Part model, mm, in its own coordinate system. A direction names the side the tool comes from. Coordinates: 2 decimals unless noted, no trailing zeros. Write each loop counter-clockwise with the first axis right and the second up, starting at its lowest first coordinate (ties: lowest second). Pieces come first, ordered by that corner, then holes. Notation, with made-up numbers: (70, 82) - (114, 82) arc R21 cw to (114, 95) - close; hole circle Ø2 at (11.5, -22.75). An arc over 180 degrees is marked (long way). Write each question's results on one line, items separated by ' | '.
from build123d import *

# Parameters (mm, degrees)
BOSS_EXTRU_1_DEPTH      = 50
CONG_1_R                = 3
COQUE2_START            = 3
COQUE2_DEPTH            = 47
ESQUISSE2_W             = 40
ESQUISSE2_H             = 8
ESQUISSE2_R             = 1.5
ESQUISSE2_W_2           = 8
ESQUISSE2_H_2           = 50
ESQUISSE2_W_3           = 25
BOSS_EXTRU_3_DEPTH      = 42
ESQUISSE3_W             = 36
ESQUISSE3_H             = 25
ENL_V_MAT_EXTRU_1_DEPTH = 10
ESQUISSE5_R             = 6.5
ENL_V_MAT_EXTRU_2_DEPTH = 10
ESQUISSE6_R             = 5.5
ENL_V_MAT_EXTRU_3_DEPTH = 10
ESQUISSE7_W             = 12
ESQUISSE7_H             = 12
ENL_V_MAT_EXTRU_4_DEPTH = 10


# Read off the part's stored shape, not the designer's step: Coque2
with BuildPart() as part:
    # Esquisse1 → Boss.-Extru.1 (new body)
    with BuildSketch(Plane(origin=(0, 0, 0), x_dir=(0, 0, -1), z_dir=(1, 0, 0))):
        Polygon((0, 0), (70, 0), (70, 140), (120, 140), (120, 230), (-30, 230), (-30, 140), (0, 140), align=None)
    extrude(amount=BOSS_EXTRU_1_DEPTH)

    # Congé1
    cong_1_edges = [part.edges().sort_by_distance(p)[0] for p in [
        (0, 140, -95),
        (0, 70, -70),
        (0, 0, -35),
        (0, 70, 0),
        (50, 70, -70),
        (25, 140, 0),
        (25, 140, 30),
        (25, 230, 30),
        (25, 230, -120),
        (25, 140, -120),
        (25, 140, -70),
        (25, 0, -70),
        (25, 0, 0),
        (50, 140, -95),
        (50, 185, -120),
        (50, 230, -45),
        (50, 185, 30),
        (50, 140, 15),
        (50, 70, 0),
        (0, 140, 15),
        (50, 0, -35),
        (0, 185, 30),
        (0, 230, -45),
        (0, 185, -120),
    ]]
    fillet(cong_1_edges, radius=CONG_1_R)

    # Coque2 outline → Coque2 (cut)
    with BuildSketch(Plane.YZ.offset(COQUE2_START)):
        with BuildLine():
            Line((137, -3), (3, -3))
            Line((3, -3), (3, -67))
            Line((3, -67), (137, -67))
            ThreePointArc((137, -67), (141.242640687, -68.757359313), (143, -73))
            Line((143, -73), (143, -117))
            Line((143, -117), (227, -117))
            Line((227, -117), (227, 27))
            Line((227, 27), (143, 27))
            Line((143, 27), (143, 3))
            ThreePointArc((143, 3), (141.242640687, -1.242640687), (137, -3))
        make_face()
    extrude(amount=COQUE2_DEPTH, mode=Mode.SUBTRACT)

    # Esquisse2 → Boss.-Extru.3 (add)
    # profile 1 of 4: a face of its own
    with BuildSketch(Plane(origin=(3, 0, 0), x_dir=(0, 0, -1), z_dir=(1, 0, 0))):
        with Locations((65, 223)):
            Rectangle(ESQUISSE2_W, ESQUISSE2_H)
        with Locations(Location((65, 223, 0), (0, 0, 180))):
            Circle(ESQUISSE2_R, mode=Mode.SUBTRACT)
    # profile 2 of 4: a face of its own
    with BuildSketch(Plane(origin=(3, 0, 0), x_dir=(0, 0, -1), z_dir=(1, 0, 0))):
        with Locations((7, 60)):
            Rectangle(ESQUISSE2_W_2, ESQUISSE2_H_2)
        with Locations(Location((7, 60, 0), (0, 0, 180))):
            Circle(ESQUISSE2_R, mode=Mode.SUBTRACT)
    # profile 3 of 4: a face of its own
    with BuildSketch(Plane(origin=(3, 0, 0), x_dir=(0, 0, -1), z_dir=(1, 0, 0))):
        with Locations((63, 60)):
            Rectangle(ESQUISSE2_W_2, ESQUISSE2_H_2)
        with Locations(Location((63, 60, 0), (0, 0, 180))):
            Circle(ESQUISSE2_R, mode=Mode.SUBTRACT)
    # profile 4 of 4: a face of its own
    with BuildSketch(Plane(origin=(3, 0, 0), x_dir=(0, 0, -1), z_dir=(1, 0, 0))):
        with Locations((25, 7)):
            Rectangle(ESQUISSE2_W_3, ESQUISSE2_H)
        with Locations(Location((25, 7, 0), (0, 0, 180))):
            Circle(ESQUISSE2_R, mode=Mode.SUBTRACT)
    extrude(amount=BOSS_EXTRU_3_DEPTH)

    # Esquisse3 → Enlèv. mat.-Extru.1 (cut)
    with BuildSketch(Plane.XY.offset(30)):
        with Locations((25, 195)):
            Rectangle(ESQUISSE3_W, ESQUISSE3_H)
    extrude(amount=-ENL_V_MAT_EXTRU_1_DEPTH, mode=Mode.SUBTRACT)

    # Esquisse5 → Enlèv. mat.-Extru.2 (cut)
    with BuildSketch(Plane.XY.offset(30)):
        with Locations((26, 161)):
            Circle(ESQUISSE5_R)
    extrude(amount=-ENL_V_MAT_EXTRU_2_DEPTH, mode=Mode.SUBTRACT)

    # Esquisse6 → Enlèv. mat.-Extru.3 (cut)
    with BuildSketch(Plane(origin=(0, 0, -70), x_dir=(-1, 0, 0), z_dir=(0, 0, -1))):
        with Locations((-25, 93)):
            Circle(ESQUISSE6_R)
    extrude(amount=-ENL_V_MAT_EXTRU_3_DEPTH, mode=Mode.SUBTRACT)

    # Esquisse7 → Enlèv. mat.-Extru.4 (cut)
    with BuildSketch(Plane(origin=(0, 0, -120), x_dir=(-1, 0, 0), z_dir=(0, 0, -1))):
        with Locations((-25, 184.5)):
            Rectangle(ESQUISSE7_W, ESQUISSE7_H)
    extrude(amount=-ENL_V_MAT_EXTRU_4_DEPTH, mode=Mode.SUBTRACT)


solid = part.part
(1) Saw through at C-C on x = 25. Count the separate pieces of the cut face and the enclosed holes in it, then the cut area to 3 significant figures.
Return value:
separate pieces: 4 | enclosed holes: 4 | area: 3,330 mm^2
(2) Saw through at A-A on y = 93. Write the cut outline in (x, z), then the cut area to 3 significant figures.
Return value:
outline: (0, -67) arc R3 ccw to (3, -70) - (19.5, -70) - (19.5, -67) - (3, -67) - (3, -3) - (50, -3) arc R3 ccw to (47, 0) - (3, 0) arc R3 ccw to (0, -3) - close; (30.5, -70) - (47, -70) arc R3 ccw to (50, -67) - (30.5, -67) - close | area: 451 mm^2
(3) Wall check: line 1 (Z direction, x = 30, y = 60); line 2 (Y direction, x = 19, z = -25); line 3 (Z direction, x = 24, y = 7). Give the ranges that are in metal, low to high. Write a range as from..to.
Return value:
line 1: z = -70..-64.5, -61.5..-59, -11..-8.5, -5.5..0 | line 2: y = 0..5.5, 8.5..11, 227..230 | line 3: z = -70..-67, -37.5..-26.5, -23.5..-12.5, -3..0
(4) 3-axis set-ups, long thin cutter, end or side, ignore diameter. For faces 5 (the flat face through (25, 140, -95)), 6 (the cylindrical face through (24.591, 154.655, 28.521)), 7 (the flat face through (24, 85, -7)): which of +Z, -Z, +X, -X, +Y, -Y reach the whole face in a straight line?
Return value:
face 5: -Z, +X, -X, -Y | face 6: +Z | face 7: +X
(5) Flat gauge pins, fed straight in: P1, Ø9, axis at x = 25, y = 93, coming from the -Z side; P2, Ø2, axis at x = 8, y = 43.5, coming from the -Z side; P3, Ø4, axis at x = 27, y = 9, coming from the +Z side. Where does each tip first touch, or does it go through?
Return value:
P1: stops at z = -3 | P2: stops at z = -70 | P3: stops at z = 0
(6) Two-plate mould, pull along Z, no slides. Class faces 1 (the flat face through (25, 176, 30)), 2 (the flat face through (26, 143, 15)), 3 (the flat face through (25, 69, -70)), 4 (the flat face through (0, 141, -44)): released by +Z, released by -Z, zero draft, split by the parting line, or undercut.
Return value:
face 1: released by +Z | face 2: undercut | face 3: released by -Z | face 4: zero draft
(7) Saw through at B-B on z = -93. Write the cut outline in (x, y), then the cut area to 3 significant figures.
Return value:
outline: (0, 143) arc R3 ccw to (3, 140) - (47, 140) arc R3 ccw to (50, 143) - (3, 143) - (3, 227) - (50, 227) arc R3 ccw to (47, 230) - (3, 230) arc R3 ccw to (0, 227) - close | area: 544 mm^2
